Here's how the part is built. I have some questions about the finished solid (model axes, mm). A direction names the side the tool comes from. Coordinates: 2 decimals unless noted, no trailing zeros. Write each loop counter-clockwise with the first axis right and the second up, starting at its lowest first coordinate (ties: lowest second). Pieces come first, ordered by that corner, then holes. Notation, with made-up numbers: (42, 81.5) - (69, 81.5) arc R17 cw to (69, 114.5) - close; hole circle Ø10 at (84, 61.25). An arc over 180 degrees is marked (long way). Answer in a Markdown table with one row per item. Add a question column.
Item 1: Imagine slicing it at B-B (z = -59.5). Please give me the cut outline in (x, y), plus the area to 3 significant figures.
Item 2: I'm going to push flat-ended pins straight in: pin 1 (2 mm diameter, centred on x = 5.5, z = -58.5, fed in from -Y); pin 2 (12 mm diameter, centred on x = 9, z = -59.5, fed in from -Y); pin 3 (4 mm diameter, centred on x = 10.5, z = -67.5, fed in from -Y). Where does each tip first touch, or does it pass through?
Item 3: Which directions (+Z, -Z, +X, -X, +Y, -Y) give clear straight access to the entire face, cutting with the end or side of a thin tool? Please do faces 1 (the face through (4, 11, 0)), 2 (the face through (-13.8, 8.1, 6.9)).
Item 4: Imagine slicing it at A-A (z = 5). Please give me the cut outline in (x, y), plus the area to 3 significant figures.
Item 5: If I drill on probe 1 along Y at (x, z) = (0, -35.5); probe 2 along Z at (x, y) = (-9, 8); probe 3 along Y at (x, z) = (11, 2.5), over which ranges is the centre line in solid material (lowest first)? Write a range as from..to.
from build123d import *

# Parameters (mm, degrees)
F1_DEPTH = 14
F4_R     = 11
F5_DEPTH = 80
F6_SIZE  = 2


with BuildPart() as f1:
    # F0 (on Top) → F1 (new body)
    with BuildSketch(Plane.XY):
        Polygon((18.475209, 0), (9.237604, 16), (-9.237604, 16), (-18.475209, 0), (-9.237604, -16), (9.237604, -16), align=None)
    extrude(amount=F1_DEPTH)

    # F2 (on Right) → F3 (revolve, cut)
    with BuildSketch(Plane.YZ):
        Polygon((-29.047782, 6.46686), (-16, 14), (-29.047782, 14), align=None)
    revolve(axis=Axis((0, 0, 10.077371), (0, 0, 1)), mode=Mode.SUBTRACT)

    # F4 (on face) → F5 (join)
    with BuildSketch(Plane(origin=(0, 0, 0), x_dir=(1, 0, 0), z_dir=(0, 0, -1))):
        Circle(F4_R)
    extrude(amount=F5_DEPTH)

    # F6
    f6_edges = [f1.edges().sort_by_distance(p)[0] for p in [
        (-11, 0, -80),
    ]]
    chamfer(f6_edges, length=F6_SIZE)


solid = f1.part
Here are the results:
| question | item | result |
|---|---|---|
| 1 | outline | circle Ø22 at (0, 0) |
| 1 | area | 380 mm2 |
| 2 | pin 1 | stops at y = -10.04 |
| 2 | pin 2 | stops at y = -10.58 |
| 2 | pin 3 | stops at y = -6.98 |
| 3 | face 1 | -Z |
| 3 | face 2 | +Z, -Z, -X, +Y |
| 4 | outline | (-18.48, 0) - (-9.24, -16) - (9.24, -16) - (18.48, 0) - (9.24, 16) - (-9.24, 16) - close |
| 4 | area | 887 mm2 |
| 5 | probe 1 | y = -11..11 |
| 5 | probe 2 | z = 0..14 |
| 5 | probe 3 | y = -12.95..12.95 |
